```python
from build123d import *

# Parameters (mm, degrees)
SKETCH1_R                  = 15
SKETCH1_R_2                = 5
BOSS_EXTRUDE1_DEPTH        = 5.8
M2_CLEARANCE_HOLE1_D       = 2.4
M2_CLEARANCE_HOLE1_DEPTH   = 25.4
M2_CLEARANCE_HOLE1_TIP     = 0.721032743
M1_6_CLEARANCE_HOLE1_D     = 1.8
M1_6_CLEARANCE_HOLE1_DEPTH = 25.4
M1_6_CLEARANCE_HOLE1_TIP   = 0.540774557
SKETCH8_W                  = 6
SKETCH8_H                  = 6
CUT_EXTRUDE1_DEPTH         = 22.99181666
FILLET1_R                  = 1
M2X0_4_TAPPED_HOLE1_D      = 1.6
M2X0_4_TAPPED_HOLE1_DEPTH  = 5.99948
M2X0_4_TAPPED_HOLE1_TIP    = 0.480688495
M2X0_4_TAPPED_HOLE2_D      = 1.6
M2X0_4_TAPPED_HOLE2_DEPTH  = 5.99948
M2X0_4_TAPPED_HOLE2_TIP    = 0.480688495


with BuildPart() as part:
    # Sketch1 → Boss-Extrude1 (new body)
    with BuildSketch(Plane.XY):
        Circle(SKETCH1_R)
        Circle(SKETCH1_R_2, mode=Mode.SUBTRACT)
    extrude(amount=BOSS_EXTRUDE1_DEPTH)

    # M2 Clearance Hole1
    with Locations(Plane.XY.offset(5.8)):
        with Locations((-11, 0), (11, 0)):
            Hole(M2_CLEARANCE_HOLE1_D / 2, depth=M2_CLEARANCE_HOLE1_DEPTH)
            with Locations((0, 0, -(M2_CLEARANCE_HOLE1_DEPTH + M2_CLEARANCE_HOLE1_TIP / 2))):  # 118° drill point
                Cone(0, M2_CLEARANCE_HOLE1_D / 2, M2_CLEARANCE_HOLE1_TIP, mode=Mode.SUBTRACT)

    # M1.6 Clearance Hole1
    with Locations(Plane.XY.offset(5.8)):
        with Locations((5.303300859, 5.303300859), (-5.303300859, -5.303300859)):
            Hole(M1_6_CLEARANCE_HOLE1_D / 2, depth=M1_6_CLEARANCE_HOLE1_DEPTH)
            with Locations((0, 0, -(M1_6_CLEARANCE_HOLE1_DEPTH + M1_6_CLEARANCE_HOLE1_TIP / 2))):  # 118° drill point
                Cone(0, M1_6_CLEARANCE_HOLE1_D / 2, M1_6_CLEARANCE_HOLE1_TIP, mode=Mode.SUBTRACT)

    # Sketch8 → Cut-Extrude1 (cut, through all)
    with BuildSketch(Plane.XY.offset(5.8)):
        with Locations((0, -12)):
            Rectangle(SKETCH8_W, SKETCH8_H)
        with Locations((0, 12)):
            Rectangle(SKETCH8_W, SKETCH8_H)
    extrude(amount=-CUT_EXTRUDE1_DEPTH, mode=Mode.SUBTRACT)

    # Fillet1
    fillet1_edges = [part.edges().sort_by_distance(p)[0] for p in [
        (-3, -14.696938457, 2.9),
        (3, -14.696938457, 2.9),
        (3, -9, 2.9),
        (-3, -9, 2.9),
        (-3, 14.696938457, 2.9),
        (3, 14.696938457, 2.9),
        (-3, 9, 2.9),
        (3, 9, 2.9),
    ]]
    fillet(fillet1_edges, radius=FILLET1_R)

    # M2x0.4 Tapped Hole1
    with Locations(Plane.XY.offset(5.8)):
        with Locations((-4.398155541, 8.448778186), (4.398155541, -8.448778186)):
            Hole(M2X0_4_TAPPED_HOLE1_D / 2, depth=M2X0_4_TAPPED_HOLE1_DEPTH)
            with Locations((0, 0, -(M2X0_4_TAPPED_HOLE1_DEPTH + M2X0_4_TAPPED_HOLE1_TIP / 2))):  # 118° drill point
                Cone(0, M2X0_4_TAPPED_HOLE1_D / 2, M2X0_4_TAPPED_HOLE1_TIP, mode=Mode.SUBTRACT)

    # M2x0.4 Tapped Hole2
    with Locations(Plane(origin=(0, 0, 0), x_dir=(-1, 0, 0), z_dir=(0, 0, -1))):
        with Locations((9.051784123, -5.22605), (-9.051784123, -5.22605), (0, 10.4521)):
            Hole(M2X0_4_TAPPED_HOLE2_D / 2, depth=M2X0_4_TAPPED_HOLE2_DEPTH)
            with Locations((0, 0, -(M2X0_4_TAPPED_HOLE2_DEPTH + M2X0_4_TAPPED_HOLE2_TIP / 2))):  # 118° drill point
                Cone(0, M2X0_4_TAPPED_HOLE2_D / 2, M2X0_4_TAPPED_HOLE2_TIP, mode=Mode.SUBTRACT)


solid = part.part
```
Here's how the part is built. I have some questions about the finished solid (model axes, mm). A direction names the side the tool comes from. Coordinates: 2 decimals unless noted, no trailing zeros. Order: outer loops, then holes, each group sorted by start corner. A loop starts at its lowest first (then second) coordinate and runs counter-clockwise, first axis right, second up. Notation, with made-up numbers: (10.5, 2.25) -> (44.5, 2.25) arc R18 ccw to (44.5, 37.25) -> close; hole circle Ø6 at (12, 21). An arc over 180 degrees is marked (long way). Return JSON: item names as keys, results as strings.
1) I'm going to push flat-ended pins straight in: P1, Ø1.7, axis at y = -11, z = 2.5, coming from the -X side; P2, Ø1.5, axis at y = 10, z = 3.5, coming from the -X side; P3, Ø1.7, axis at y = 12.5, z = 2.5, coming from the -X side; P4, Ø1.4, axis at x = 9.05, y = -5.23, coming from the +Z side. Where does each tip first touch, or does it pass through?
Conclusion:
{"P1": "stops at x = -11.04", "P2": "stops at x = -11.81", "P3": "stops at x = -9.45", "P4": "passes through"}
2) If we section it at A-A on x = 0: List the corners of the cut face in (y, z) for me.
Conclusion:
{"outline": "(-9, 0) -> (-5, 0) -> (-5, 5.8) -> (-9, 5.8) -> close; (5, 0) -> (9, 0) -> (9, 5.8) -> (5, 5.8) -> close"}
3) If we section it at B-B on y = 0: List the corners of the cut face in (x, z) for me, plus the area to 3 significant figures.
Conclusion:
{"outline": "(-15, 0) -> (-12.2, 0) -> (-12.2, 5.8) -> (-15, 5.8) -> close; (-9.8, 0) -> (-5, 0) -> (-5, 5.8) -> (-9.8, 5.8) -> close; (5, 0) -> (9.8, 0) -> (9.8, 5.8) -> (5, 5.8) -> close; (12.2, 0) -> (15, 0) -> (15, 5.8) -> (12.2, 5.8) -> close", "area": "88.2 mm²"}
4) If we section it at C-C on z = 2.95: State how many separate pieces and enclosed holes the cut face has, plus the area to 3 significant figures.
Conclusion:
{"separate pieces": "1", "enclosed holes": "9", "area": "535 mm²"}
5) Thinking about a two-plate mould opening in X: for faces 4 (the cylindrical face through (15, 0, 3)), 5 (the cylindrical face through (5.03, -8.94, 2.86)), 6 (the cylindrical face through (-15, 0, 3)), which applies, +X half, -X half, draft (parallel to the pull), parting line (faces both ways), or undercut?
Conclusion:
{"face 4": "+X half", "face 5": "undercut", "face 6": "-X half"}
6) On a 3-axis mill with a long thin cutter (end or side, diameter ignored), from which of +Z, -Z, +X, -X, +Y, -Y can I reach the whole of each face in a straight line? I mean faces 1 (the cylindrical face through (2.699, -9.285, 2.859)), 2 (the cylindrical face through (-3.6, 8.5, 2.9)), 3 (the flat face through (3, 12, 3)). Say none if no direction works.
Conclusion:
{"face 1": "+Z, -Z, -Y", "face 2": "+Z, -Z", "face 3": "+Z, -Z, +Y"}
7) If I drill on probe 1 along Y at (x, z) = (4, 4.8); probe 2 along Y at (x, z) = (-10.75, 0.65); probe 3 along Y at (x, z) = (11, 4.25), over which ranges is the centre line in solid material (lowest first)?
Conclusion:
{"probe 1": "y = -14.42 to -9.14, -7.75 to -3, 3 to 14.42", "probe 2": "y = -10.46 to -1.17, 1.17 to 10.46", "probe 3": "y = -10.2 to -1.2, 1.2 to 10.2"}
8) If we section it at D-D on x = -11.25: List the corners of the cut face in (y, z) for me.
Conclusion:
{"outline": "(-9.92, 0) -> (-1.17, 0) -> (-1.17, 5.8) -> (-9.92, 5.8) -> close; (1.17, 0) -> (9.92, 0) -> (9.92, 5.8) -> (1.17, 5.8) -> close"}
